```python
from build123d import *

# Parameters (mm, degrees)
F1_DEPTH = 29
F2_W     = 155.196704
F2_H     = 36
F3_DEPTH = 11
F5_DEPTH = 27.001
F6_R     = 3


with BuildPart() as f1:
    # F0 (on Front) → F1 (new body, symmetric)
    with BuildSketch(Plane.XZ):
        with BuildLine():
            Line((34.5, 19), (-34.5, 19))
            ThreePointArc((-34.5, 19), (-55.006097, 10.506097), (-63.5, -10))
            Line((-63.5, -10), (-63.5, -13))
            Line((-63.5, -13), (-52.5, -13))
            Line((-52.5, -13), (-52.5, -19))
            Line((-52.5, -19), (52.5, -19))
            Line((52.5, -19), (52.5, -13))
            Line((52.5, -13), (63.5, -13))
            Line((63.5, -13), (63.5, -10))
            ThreePointArc((63.5, -10), (55.006097, 10.506097), (34.5, 19))
        make_face()
    extrude(amount=F1_DEPTH, both=True)

    # F2 (on face) → F3 (cut)
    with BuildSketch(Plane.XY.offset(19)):
        with Locations((-5.67447, 0)):
            Rectangle(F2_W, F2_H)
    extrude(amount=-F3_DEPTH, mode=Mode.SUBTRACT)

    # F4 (on face) → F5 (cut, through all)
    with BuildSketch(Plane.XY.offset(8)):
        with BuildLine():
            Line((-24.237634, 6.5), (-43.237634, 6.5))
            ThreePointArc((-43.237634, 6.5), (-49.737634, 0), (-43.237634, -6.5))
            Line((-43.237634, -6.5), (-24.237634, -6.5))
            ThreePointArc((-24.237634, -6.5), (-17.737634, 0), (-24.237634, 6.5))
        make_face()
        with BuildLine():
            Line((43.237634, 6.5), (24.237634, 6.5))
            ThreePointArc((24.237634, 6.5), (17.737634, 0), (24.237634, -6.5))
            Line((24.237634, -6.5), (43.237634, -6.5))
            ThreePointArc((43.237634, -6.5), (49.737634, 0), (43.237634, 6.5))
        make_face()
    extrude(amount=-F5_DEPTH, mode=Mode.SUBTRACT)

    # F6
    f6_edges = [f1.edges().sort_by_distance(p)[0] for p in [
        (-55.006097, -29, 10.506097),
        (55.006097, 29, 10.506097),
    ]]
    fillet(f6_edges, radius=F6_R)


solid = f1.part
```
Input: part model. Units: mm. Frame: model coordinates. A direction names the side the tool comes from. Coordinates: 2 decimals unless noted, no trailing zeros. Write each loop counter-clockwise with the first axis right and the second up, starting at its lowest first coordinate (ties: lowest second). Pieces come first, ordered by that corner, then holes. Notation, with made-up numbers: M -5,-39.75 L 31,-39.75 A26 ccw 31,-12.75 Z; hole C -11.75,41.25 d3. An arc over 180 degrees is marked long. Use one line per item in the form item = value.
Q1. Draft query along Y for faces 6 (the face through (-1, -18, 14)), 7 (the face through (62.64, 28.1, -11.48)), 8 (the face through (-34, -6.5, -5)), 9 (the face through (-1, 0, -19)). Return one class per face: released by +Y, released by -Y, zero draft, split by the parting line, or undercut.
Answer below:
face_6 = undercut
face_7 = released by +Y
face_8 = undercut
face_9 = zero draft
Q2. Section C-C (z = -14.5). Return loops of the section in (x, y), plus the area to 3 significant figures.
Answer below:
outline = M -52.5,-29 L 52.5,-29 L 52.5,29 L -52.5,29 Z; hole M -43.24,-6.5 L -24.24,-6.5 A6.5 ccw -24.24,6.5 L -43.24,6.5 A6.5 ccw Z; hole M 24.24,-6.5 L 43.24,-6.5 A6.5 ccw 43.24,6.5 L 24.24,6.5 A6.5 ccw Z
area = 5,330 mm²
Q3. Section A-A (y = 0). Return loops of the section in (x, z).
Answer below:
outline = M -63.5,-13 L -52.5,-13 L -52.5,-19 L -49.74,-19 L -49.74,8 L -57.24,8 A29 ccw -63.5,-10 Z; M -17.74,-19 L 17.74,-19 L 17.74,8 L -17.74,8 Z; M 49.74,-19 L 52.5,-19 L 52.5,-13 L 63.5,-13 L 63.5,-10 A29 ccw 57.24,8 L 49.74,8 Z
Q4. Section B-B (x = 4.5). Return loops of the section in (y, z), plus the area to 3 significant figures.
Answer below:
outline = M -29,-19 L 29,-19 L 29,16 A3 ccw 26,19 L 18,19 L 18,8 L -18,8 L -18,19 L -26,19 A3 ccw -29,16 Z
area = 1,800 mm²
Q5. Material intervals for probe 1 along Y at (x, z) = (30, -1.5); probe 2 along Y at (x, z) = (30, 8.5); probe 3 along X at (y, z) = (2, -10.5), sorted ascending. Write a range as from..to.
Answer below:
probe_1 = -29..-6.5, 6.5..29
probe_2 = -29..-18, 18..29
probe_3 = -63.5..-49.42, -18.05..18.05, 49.42..63.5
Q6. Section D-D (x = 25.5). Return loops of the section in (y, z).
Answer below:
outline = M -29,-19 L -6.5,-19 L -6.5,8 L -18,8 L -18,19 L -26,19 A3 ccw -29,16 Z; M 6.5,-19 L 29,-19 L 29,16 A3 ccw 26,19 L 18,19 L 18,8 L 6.5,8 Z
Q7. Set-up query: faces 1 (the face through (-52.5, 0, -16)), 2 (the face through (-1, 0, 8)), 3 (the face through (34, 6.5, -5)), 4 (the face through (58, 0, -13)), 5 (the face through (-60.65, -0.36, 2.54)). Return all of +Z, -Z, +X, -X, +Y, -Y with unobstructed straight access to the full face (end or side cutting, diameter ignored); none if empty.
Answer below:
face_1 = -Z, -X, +Y, -Y
face_2 = +Z, +X, -X
face_3 = +Z, -Z
face_4 = -Z, +X, +Y, -Y
face_5 = +Z, -X, +Y, -Y
Q8. First-contact query: pin 1 (6 mm diameter, centred on y = -8, z = -14.5, fed in from -X); pin 2 (3.5 mm diameter, centred on x = -57, y = -7, fed in from -Z); pin 3 (1 mm diameter, centred on x = -23, y = 8, fed in from +Z); pin 4 (3 mm diameter, centred on y = 13.5, z = -15, fed in from +X). Flat tips, straight axial feed; report the tip coordinate or a pass-through.
Answer below:
pin_1 = -63.5
pin_2 = -13
pin_3 = 8
pin_4 = 52.5
